Autodesk Fusion 360 part; units mm, degrees
sketch "Sketch1" plane through (0, 0, 0) normal (0, 0, 1) x (1, 0, 0)
  line L0 (22.1, 35.95) -> (-22.1, 35.95) construction
  line L1 (-22.1, 35.95) -> (-22.1, -35.95) construction
  line L2 (-22.1, -35.95) -> (22.1, -35.95) construction
  line L3 (22.1, -35.95) -> (22.1, 35.95) construction
  line L4 (22.1, 35.95) -> (-22.1, -35.95) construction
  line L5 (-22.1, 35.95) -> (22.1, -35.95) construction
  line L6 (23.8, 37.65) -> (-23.8, 37.65) construction
  line L7 (-23.8, 37.65) -> (-23.8, -37.65) construction
  line L8 (-23.8, -37.65) -> (23.8, -37.65) construction
  line L9 (23.8, -37.65) -> (23.8, 37.65) construction
  line L10 (23.8, 37.65) -> (-23.8, -37.65) construction
  line L11 (-23.8, 37.65) -> (23.8, -37.65) construction
  circle A0 centre (-22.1, 35.95) radius 1.7
  circle A1 centre (22.1, 35.95) radius 1.7
  circle A2 centre (-22.1, -35.95) radius 1.7
  circle A3 centre (22.1, -35.95) radius 1.7
  line L12 (-23.8, -34.25) -> (23.8, -34.25) construction
  line L13 (-20.4, -37.65) -> (-20.4, 37.65) construction
  line L14 (-23.8, 34.25) -> (23.8, 34.25) construction
  line L15 (20.4, 37.65) -> (20.4, -37.65) construction
  line L16 (31, 47.5) -> (-31, 47.5)
  line L17 (-31, 47.5) -> (-31, -47.5)
  line L18 (-31, -47.5) -> (31, -47.5)
  line L19 (31, -47.5) -> (31, 47.5)
  line L20 (31, 47.5) -> (-31, -47.5) construction
  line L21 (-31, 47.5) -> (31, -47.5) construction
  circle A4 centre (-45, 0) radius 3
  circle A5 centre (45, 0) radius 3
  circle A6 centre (-45, 0) radius 7.5
  circle A7 centre (45, 0) radius 7.5
  line L22 (-31, 47.5) -> (-51.7899, 3.1854)
  line L23 (-31, -47.5) -> (-51.7899, -3.1854)
  line L24 (31, -47.5) -> (51.7899, -3.1854)
  line L25 (31, 47.5) -> (51.7899, 3.1854)
  line L26 (45, 0) -> (0, 0) construction
  line L27 (0, 0) -> (-45, 0) construction
  circle A8 centre (12.1, 35.95) radius 2.5
  dimension "d1" = 75.3
  dimension "d2" = 68.5
  dimension "d3" = 40.8
  dimension "d4" = 47.6
  dimension "d5" = 95
  dimension "d6" = 62
  dimension "d7" = 6
  dimension "d8" = 6
  dimension "d9" = 15
  dimension "d10" = 15
  dimension "d11" = 45
  dimension "d12" = 45
  dimension "d13" = 10
  dimension "d14" = 5
extrude "Extrude1" add sketch "Sketch1" along normal blind 4
fillet "Fillet1" radius 5 4 edges at (31, 47.5, 2) (-31, 47.5, 2) (31, -47.5, 2) (-31, -47.5, 2)
sketch "Sketch2" plane through (0, 0, 0) normal (0, 0, -1) x (1, 0, 0)
  circle A0 centre (45, 0) radius 3
  circle A1 centre (-22.1, 35.95) radius 1.7
  circle A2 centre (22.1, 35.95) radius 1.7
  circle A3 centre (-22.1, -35.95) radius 1.7
  circle A4 centre (-45, 0) radius 3
  circle A5 centre (22.1, -35.95) radius 1.7
  circle A6 centre (12.1, -35.95) radius 2.5
  arc A7 (-27.8228, 47.5) -> (-32.3494, 44.6236) centre (-27.8228, 42.5) ccw
  line L0 (-32.3494, 44.6236) -> (-51.7899, 3.1854)
  arc A8 (-51.7899, 3.1854) -> (-51.7899, -3.1854) centre (-45, 0) ccw
  line L1 (-51.7899, -3.1854) -> (-32.3494, -44.6236)
  arc A9 (-32.3494, -44.6236) -> (-27.8228, -47.5) centre (-27.8228, -42.5) ccw
  line L2 (-27.8228, -47.5) -> (27.8228, -47.5)
  arc A10 (27.8228, -47.5) -> (32.3494, -44.6236) centre (27.8228, -42.5) ccw
  line L3 (32.3494, -44.6236) -> (51.7899, -3.1854)
  arc A11 (51.7899, -3.1854) -> (51.7899, 3.1854) centre (45, 0) ccw
  line L4 (51.7899, 3.1854) -> (32.3494, 44.6236)
  arc A12 (32.3494, 44.6236) -> (27.8228, 47.5) centre (27.8228, 42.5) ccw
  line L5 (27.8228, 47.5) -> (-27.8228, 47.5)
  circle A13 centre (22.1, -35.95) radius 4.25
  circle A14 centre (-22.1, -35.95) radius 4.25
  circle A15 centre (-22.1, 35.95) radius 4.25
  circle A16 centre (22.1, 35.95) radius 4.25
  dimension "d19" = 8.5
  dimension "d20" = 8.5
  dimension "d21" = 8.5
  dimension "d22" = 8.5
extrude "Extrude2" cut sketch "Sketch2" against normal blind 2.4 contours A13 | A14 | A15 | A16
sketch "Sketch3" plane through (0, 0, 4) normal (0, 0, 1) x (-1, 0, 0)
  arc A0 (32.3494, 44.6236) -> (27.8228, 47.5) centre (27.8228, 42.5) ccw
  line L0 (27.8228, 47.5) -> (-27.8228, 47.5)
  arc A1 (-27.8228, 47.5) -> (-32.3494, 44.6236) centre (-27.8228, 42.5) ccw
  line L1 (-32.3494, 44.6236) -> (-51.7899, 3.1854)
  arc A2 (-51.7899, 3.1854) -> (-51.7899, -3.1854) centre (-45, 0) ccw
  line L2 (-51.7899, -3.1854) -> (-32.3494, -44.6236)
  arc A3 (-32.3494, -44.6236) -> (-27.8228, -47.5) centre (-27.8228, -42.5) ccw
  line L3 (-27.8228, -47.5) -> (27.8228, -47.5)
  arc A4 (27.8228, -47.5) -> (32.3494, -44.6236) centre (27.8228, -42.5) ccw
  line L4 (32.3494, -44.6236) -> (51.7899, -3.1854)
  arc A5 (51.7899, -3.1854) -> (51.7899, 3.1854) centre (45, 0) ccw
  line L5 (51.7899, 3.1854) -> (32.3494, 44.6236)
  circle A6 centre (-45, 0) radius 3
  circle A7 centre (22.1, 35.95) radius 1.7
  circle A8 centre (-22.1, 35.95) radius 1.7
  circle A9 centre (22.1, -35.95) radius 1.7
  circle A10 centre (45, 0) radius 3
  circle A11 centre (-22.1, -35.95) radius 1.7
  circle A12 centre (-12.1, -35.95) radius 2.5
  circle A13 centre (22.1, -35.95) radius 2
  circle A14 centre (-22.1, -35.95) radius 2
  circle A15 centre (-22.1, 35.95) radius 2
  circle A16 centre (22.1, 35.95) radius 2
  dimension "d25" = 4
  dimension "d26" = 4
  dimension "d27" = 4
  dimension "d28" = 4
extrude "Extrude3" cut sketch "Sketch3" against normal up to surface (1.6 mm away) contours A13 | A14 | A15 | A16
sketch "Sketch4" plane through (0, 0, 2.4) normal (0, 0, -1) x (1, 0, 0)
  circle A0 centre (-22.1, -35.95) radius 2
  circle A1 centre (-22.1, -35.95) radius 4.25
  circle A2 centre (-22.1, 35.95) radius 2
  circle A3 centre (-22.1, 35.95) radius 4.25
  circle A4 centre (22.1, 35.95) radius 2
  circle A5 centre (22.1, 35.95) radius 4.25
  circle A6 centre (22.1, -35.95) radius 2
  circle A7 centre (22.1, -35.95) radius 4.25
  line L0 (-24.1, 39.7) -> (-24.1, 32.2)
  line L1 (-20.1, 39.7) -> (-20.1, 32.2)
  line L2 (20.1, 39.7) -> (20.1, 32.2)
  line L3 (24.1, 39.7) -> (24.1, 32.2)
  line L4 (24.1, -32.2) -> (24.1, -39.7)
  line L5 (20.1, -32.2) -> (20.1, -39.7)
  line L6 (-20.1, -32.2) -> (-20.1, -39.7)
  line L7 (-24.1, -32.2) -> (-24.1, -39.7)
extrude "Extrude4" cut sketch "Sketch4" against normal blind 0.2 contours A0 A1 L6 L7 | A0 A1 L6 L7 | A2 A3 L0 L1 | A2 A3 L0 L1 | A4 A5 L2 L3 | A4 A5 L2 L3 | A6 A7 L4 L5 | A6 A7 L4 L5
sketch "Sketch5" plane through (0, 0, 2.6) normal (0, 0, -1) x (1, 0, 0)
  line L0 (-24.1, 39.7) -> (-24.1, 35.95)
  arc A0 (-20.1, 35.95) -> (-24.1, 35.95) centre (-22.1, 35.95) ccw
  line L1 (-20.1, 35.95) -> (-20.1, 39.7)
  arc A1 (-20.1, 39.7) -> (-24.1, 39.7) centre (-22.1, 35.95) ccw
  arc A2 (20.1, 32.2) -> (24.1, 32.2) centre (22.1, 35.95) ccw
  line L2 (24.1, 32.2) -> (24.1, 35.95)
  arc A3 (20.1, 35.95) -> (24.1, 35.95) centre (22.1, 35.95) ccw
  line L3 (20.1, 35.95) -> (20.1, 32.2)
  line L4 (20.1, 39.7) -> (20.1, 35.95)
  arc A4 (24.1, 35.95) -> (20.1, 35.95) centre (22.1, 35.95) ccw
  line L5 (24.1, 35.95) -> (24.1, 39.7)
  arc A5 (24.1, 39.7) -> (20.1, 39.7) centre (22.1, 35.95) ccw
  arc A6 (-24.1, 32.2) -> (-20.1, 32.2) centre (-22.1, 35.95) ccw
  line L6 (-20.1, 32.2) -> (-20.1, 35.95)
  arc A7 (-24.1, 35.95) -> (-20.1, 35.95) centre (-22.1, 35.95) ccw
  line L7 (-24.1, 35.95) -> (-24.1, 32.2)
  line L8 (20.1, -35.95) -> (20.1, -39.7)
  arc A8 (20.1, -39.7) -> (24.1, -39.7) centre (22.1, -35.95) ccw
  line L9 (24.1, -39.7) -> (24.1, -35.95)
  arc A9 (20.1, -35.95) -> (24.1, -35.95) centre (22.1, -35.95) ccw
  arc A10 (24.1, -32.2) -> (20.1, -32.2) centre (22.1, -35.95) ccw
  line L10 (20.1, -32.2) -> (20.1, -35.95)
  arc A11 (24.1, -35.95) -> (20.1, -35.95) centre (22.1, -35.95) ccw
  line L11 (24.1, -35.95) -> (24.1, -32.2)
  line L12 (-24.1, -35.95) -> (-24.1, -39.7)
  arc A12 (-24.1, -39.7) -> (-20.1, -39.7) centre (-22.1, -35.95) ccw
  line L13 (-20.1, -39.7) -> (-20.1, -35.95)
  arc A13 (-24.1, -35.95) -> (-20.1, -35.95) centre (-22.1, -35.95) ccw
  arc A14 (-20.1, -32.2) -> (-24.1, -32.2) centre (-22.1, -35.95) ccw
  line L14 (-24.1, -32.2) -> (-24.1, -35.95)
  arc A15 (-20.1, -35.95) -> (-24.1, -35.95) centre (-22.1, -35.95) ccw
  line L15 (-20.1, -35.95) -> (-20.1, -32.2)
  line L16 (-24.1, 37.95) -> (-20.1, 37.95)
  line L17 (-24.1, 33.95) -> (-20.1, 33.95)
  line L18 (20.1, 37.95) -> (24.1, 37.95)
  line L19 (20.1, 33.95) -> (24.1, 33.95)
  line L20 (20.1, -33.95) -> (24.1, -33.95)
  line L21 (24.1, -37.95) -> (20.1, -37.95)
  line L22 (-24.1, -33.95) -> (-20.1, -33.95)
  line L23 (-24.1, -37.95) -> (-20.1, -37.95)
extrude "Extrude5" cut sketch "Sketch5" against normal blind 0.2 contours L0 A0 L16 | A7 L7 L17 | A0 L1 L16 | L6 A7 L17 | A3 L3 L19 | L2 A3 L19 | L4 A4 L18 | A4 L5 L18 | L8 A9 L21 | L10 A11 L20 | L9 A9 L21 | A11 L11 L20 | L12 A13 L23 | L14 A15 L22 | L13 A13 L23 | A15 L15 L22
chamfer "Chamfer1" distance 2 angle 45 2 edges at (-47.797, 1.0848, 4) (42.203, 1.0848, 4)
Geometry: final body of the model. Coordinates: model frame, mm. A direction names the side the tool comes from. Give positions to 0.01 mm unless a question says otherwise; leave off trailing zeros. Write each loop counter-clockwise with the first axis right and the second up, starting at its lowest first coordinate (ties: lowest second). Pieces come first, ordered by that corner, then holes.
(1) Cut plane B-B, the plane x = -45. Return loops of the section in (y, z), then the cut area to 3 significant figures.
(2) Cut plane A-A, the plane y = 0. Return loops of the section in (x, z).
(3) Cut plane C-C, the plane y = 24. Return loops of the section in (x, z).
(4) Ray query, line 1 (Y direction, x = 22.1, z = 1); line 2 (X direction, y = 1.5, z = 2.95); line 3 (X direction, y = -35.95, z = 3.7). Return the intervals inside material, ascending.
(5) Access query for faces 1 (the flat face through (22, 39, 2.6)), 2 (the cylindrical face through (-23.947, -35.184, 3.408)). Directions: +Z, -Z, +X, -X, +Y, -Y. A direction counts if a zero-diameter tool reaches every point of the face in a straight line with its end or side. Return the directions, or none.
(6) First-contact query: P1, Ø1, axis at y = -27, z = 2, coming from the -X side; P2, Ø0.7, axis at x = -22.5, y = 39, coming from the -Z side; P3, Ø1, axis at x = 23, y = -35, coming from the -Z side; P4, Ø2, axis at x = -20.5, y = 35, coming from the -Z side. Flat tips, straight axial feed; report the tip coordinate or a pass-through.
Values follow:
1. outline: (-17.66, 0) - (-3, 0) - (-3, 2) - (-5, 4) - (-17.66, 4) - close; (3, 0) - (17.66, 0) - (17.66, 4) - (5, 4) - (3, 2) - close
1. area: 113 mm2
2. outline: (-52.5, 0) - (-48, 0) - (-48, 2) - (-50, 4) - (-52.5, 4) - close; (-42, 0) - (42, 0) - (42, 2) - (40, 4) - (-40, 4) - (-42, 2) - close; (48, 0) - (52.5, 0) - (52.5, 4) - (50, 4) - (48, 2) - close
3. outline: (-42.02, 0) - (42.02, 0) - (42.02, 4) - (-42.02, 4) - close
4. line 1: y = -47.5 to -40.2, -31.7 to 31.7, 40.2 to 47.5
4. line 2: x = -52.35 to -48.65, -41.35 to 41.35, 48.65 to 52.35
4. line 3: x = -36.42 to -24.1, -20.1 to 20.1, 24.1 to 36.42
5. face 1: -Z
5. face 2: +Z, -Z
6. P1: stops at x = -40.85
6. P2: stops at z = 2.6
6. P3: passes through
6. P4: stops at z = 2.4
